```python
from build123d import *

# Parameters (mm, degrees)
SKETCH1_R           = 18
SKETCH1_R_2         = 8
BOSS_EXTRUDE1_DEPTH = 8
SKETCH2_R           = 8
SKETCH2_R_2         = 6
BOSS_EXTRUDE2_DEPTH = 5.5
SKETCH3_W           = 40
SKETCH3_H           = 20
CUT_EXTRUDE1_DEPTH  = 10.5
CUT_EXTRUDE2_REACH  = 19
SKETCH5_R           = 1.6
CUT_EXTRUDE3_REACH  = 29
CUT_EXTRUDE3_START  = -10


with BuildPart() as part:
    # Sketch1 → Boss-Extrude1 (new body)
    with BuildSketch(Plane(origin=(0, 0, 0), x_dir=(1, 0, 0), z_dir=(0, 1, 0))):
        Circle(SKETCH1_R)
        Circle(SKETCH1_R_2, mode=Mode.SUBTRACT)
        with BuildLine():
            Line((-7.950852961, 12.5), (-7.950852961, 9.5))
            ThreePointArc((-7.950852961, 9.5), (-6.350852961, 7.9), (-4.750852961, 9.5))
            Line((-4.750852961, 9.5), (-4.750852961, 12.5))
            ThreePointArc((-4.750852961, 12.5), (-6.350852961, 14.1), (-7.950852961, 12.5))
        make_face(mode=Mode.SUBTRACT)
        with BuildLine():
            Line((4.750852961, 12.5), (4.750852961, 9.5))
            ThreePointArc((4.750852961, 9.5), (6.350852961, 7.9), (7.950852961, 9.5))
            Line((7.950852961, 9.5), (7.950852961, 12.5))
            ThreePointArc((7.950852961, 12.5), (6.350852961, 14.1), (4.750852961, 12.5))
        make_face(mode=Mode.SUBTRACT)
    extrude(amount=BOSS_EXTRUDE1_DEPTH)

    # Sketch2 → Boss-Extrude2 (add)
    with BuildSketch(Plane(origin=(0, 4, 0), x_dir=(1, 0, 0), z_dir=(0, 1, 0))):
        Circle(SKETCH2_R)
        Circle(SKETCH2_R_2, mode=Mode.SUBTRACT)
    extrude(amount=-BOSS_EXTRUDE2_DEPTH)

    # Sketch3 → Cut-Extrude1 (cut, through all)
    with BuildSketch(Plane(origin=(0, 8, 0), x_dir=(1, 0, 0), z_dir=(0, 1, 0))):
        with Locations((0, -9)):
            Rectangle(SKETCH3_W, SKETCH3_H)
    extrude(amount=-CUT_EXTRUDE1_DEPTH, mode=Mode.SUBTRACT)

    # Sketch5 → Cut-Extrude2 (cut, up to next)
    with BuildSketch(Plane.XY.offset(-1), mode=Mode.PRIVATE) as cut_extrude2_sk1:
        with Locations((-12.954727344, 4)):
            Circle(SKETCH5_R)
    cut_extrude2_tool1 = extrude(cut_extrude2_sk1.sketch, amount=-CUT_EXTRUDE2_REACH, mode=Mode.PRIVATE) & part.part
    add(cut_extrude2_tool1.solids().sort_by_distance((-12.954727, 4, -1))[0], mode=Mode.SUBTRACT)
    # Sketch5 → Cut-Extrude2 (cut, up to next)
    with BuildSketch(Plane.XY.offset(-1), mode=Mode.PRIVATE) as cut_extrude2_sk2:
        with Locations((12.954727344, 4)):
            Circle(SKETCH5_R)
    cut_extrude2_tool2 = extrude(cut_extrude2_sk2.sketch, amount=-CUT_EXTRUDE2_REACH, mode=Mode.PRIVATE) & part.part
    add(cut_extrude2_tool2.solids().sort_by_distance((12.954727, 4, -1))[0], mode=Mode.SUBTRACT)

    # Sketch6 → Cut-Extrude3 (cut, up to next)
    with BuildSketch(Plane.XY.offset(-1).offset(CUT_EXTRUDE3_START), mode=Mode.PRIVATE) as cut_extrude3_sk1:
        Polygon((-9.721565837, 4), (-11.338146591, 6.8), (-14.571308098, 6.8), (-16.187888852, 4), (-14.571308098, 1.2), (-11.338146591, 1.2), align=None)
    cut_extrude3_tool1 = extrude(cut_extrude3_sk1.sketch, amount=-CUT_EXTRUDE3_REACH, mode=Mode.PRIVATE) & part.part
    add(cut_extrude3_tool1.solids().sort_by_distance((-12.954727, 4, -11))[0], mode=Mode.SUBTRACT)
    # Sketch6 → Cut-Extrude3 (cut, up to next)
    with BuildSketch(Plane.XY.offset(-1).offset(CUT_EXTRUDE3_START), mode=Mode.PRIVATE) as cut_extrude3_sk2:
        Polygon((16.187888852, 4), (14.571308098, 6.8), (11.338146591, 6.8), (9.721565837, 4), (11.338146591, 1.2), (14.571308098, 1.2), align=None)
    cut_extrude3_tool2 = extrude(cut_extrude3_sk2.sketch, amount=-CUT_EXTRUDE3_REACH, mode=Mode.PRIVATE) & part.part
    add(cut_extrude3_tool2.solids().sort_by_distance((12.954727, 4, -11))[0], mode=Mode.SUBTRACT)


solid = part.part
```
Here's how the part is built. I have some questions about the finished solid (model axes, mm). A direction names the side the tool comes from. Round coordinates to 2 decimals unless told otherwise and drop trailing zeros. Write each loop counter-clockwise with the first axis right and the second up, starting at its lowest first coordinate (ties: lowest second). Pieces come first, ordered by that corner, then holes.
Q1. If we section it at C-C on y = 0.5: Write out the boundary of the cut face in (x, z), plus the area to 3 significant figures.
Q2. Please list where these lines run through material, in increasing order: probe 1 along X at (y, z) = (4, -8.5); probe 2 along Y at (x, z) = (6, -6.75); probe 3 along X at (y, z) = (0.75, -1.75).
Q3. Which directions (+Z, -Z, +X, -X, +Y, -Y) give clear straight access to the entire face, cutting with the end or side of a thin tool? Please do faces 1 (the flat face through (12, 1.2, -12)), 2 (the flat face through (-7.951, 4, -11)), 3 (the cylindrical face through (0, -1, -8)).
Q4. If we mould it in two halves opening along X, with no side actions, what happens to faces 4 (the flat face through (-12, 6.8, -12)), 5 (the cylindrical face through (0, 6, -8)), 6 (the flat face through (-10.52, 5.38, -12.58))? For each: +X half, -X half, draft (parallel to the pull), parting line (faces both ways), or undercut.
Q5. If we section it at B-B on x = -12.5: Write out the boundary of the cut face in (y, z), plus the area to 3 significant figures.
Q6. Will these pins go through, and if not, where does the flat tip stop? P1, Ø3.5, axis at x = 2.5, z = -5, coming from the +Y side; P2, Ø3, axis at x = -12.95, y = 4, coming from the -Z side (3 decimals); P3, Ø5, axis at x = 14, z = -5, coming from the -Y side; P4, Ø1.5, axis at y = 7, z = -3.5, coming from the -X side.
Q7. If we section it at D-D on x = 0: Write out the boundary of the cut face in (y, z).
Q8. If we section it at A-A on z = -4.25: Write out the boundary of the cut face in (x, y), plus the area to 3 significant figures.
Answer below:
1. outline: (-17.97, -1) arc R18 ccw to (17.97, -1) - (5.92, -1) arc R6 cw to (-5.92, -1) - close; hole (-7.95, -12.5) arc R1.6 ccw to (-4.75, -12.5) - (-4.75, -9.5) arc R1.6 ccw to (-7.95, -9.5) - close; hole (4.75, -12.5) arc R1.6 ccw to (7.95, -12.5) - (7.95, -9.5) arc R1.6 ccw to (4.75, -9.5) - close
1. area: 393 mm2
2. probe 1: x = -15.87 to -14.55, -11.35 to -7.6, -5.1 to 5.1, 7.6 to 11.35, 14.55 to 15.87
2. probe 2: y = 0 to 8
2. probe 3: x = -17.91 to -5.74, 5.74 to 17.91
3. face 1: -Z, +X
3. face 2: +Y, -Y
3. face 3: -Z, -Y
4. face 4: draft
4. face 5: undercut
4. face 6: -X half
5. outline: (0, -12.95) - (1.2, -12.95) - (1.2, -11) - (2.47, -11) - (2.47, -1) - (0, -1) - close; (5.53, -11) - (6.8, -11) - (6.8, -12.95) - (8, -12.95) - (8, -1) - (5.53, -1) - close
5. area: 54.0 mm2
6. P1: stops at y = 4
6. P2: passes through
6. P3: stops at y = 0
6. P4: stops at x = -17.79
7. outline: (-1.5, -8) - (0, -8) - (0, -18) - (8, -18) - (8, -8) - (4, -8) - (4, -6) - (-1.5, -6) - close
8. outline: (-17.49, 0) - (-6.78, 0) - (-6.78, -1.5) - (-4.24, -1.5) - (-4.24, 4) - (-6.78, 4) - (-6.78, 8) - (-17.49, 8) - close; (4.24, -1.5) - (6.78, -1.5) - (6.78, 0) - (17.49, 0) - (17.49, 8) - (6.78, 8) - (6.78, 4) - (4.24, 4) - close; hole circle Ø3.2 at (-12.95, 4); hole circle Ø3.2 at (12.95, 4)
8. area: 183 mm2
